Geometry: final body of the model. Coordinates: model frame, mm. A direction names the side the tool comes from. Give positions to 0.01 mm unless a question says otherwise; leave off trailing zeros. Answer as a JSON object with one key per item and string values. Group by question number.
(1) Material intervals for probe 1 along Z at (x, y) = (24.5, 5); probe 2 along Z at (x, y) = (31.5, 4); probe 3 along Y at (x, z) = (4, 50.5), sorted ascending.
(2) Set-up query: faces 1 (the face through (-1, 0, 6.35)), 2 (the face through (38.1, 0, 66)). Return all of +Z, -Z, +X, -X, +Y, -Y with unobstructed straight access to the full face (end or side cutting, diameter ignored); none if empty.
(3) Contact query for flat-ended pins moving along their axis: pin 1 Ø6 at (y, z) = (-5, 24) entering from -X; pin 2 Ø1.5 at (x, y) = (9.5, -3) entering from +Z; pin 3 Ø2 at (x, y) = (10, -1.5) entering from +Z. Output: stop coordinate, or through.
from build123d import *

# Parameters (mm, degrees)
F1_DEPTH = 6.35
F2_R     = 5.08


with BuildPart() as f1:
    # F0 (on Front) → F1 (new body, symmetric)
    with BuildSketch(Plane.XZ):
        with BuildLine():
            Line((-63.5, 6.35), (63.5, 6.35))
            add(Edge.make_bspline(
                [(63.5, 6.35), (-38.796838, 20.9835), (10.021353, 59.327461), (38.1, 59.931301)],
                knots=[0, 0, 0, 0, 59.296845, 59.296845, 59.296845, 59.296845], degree=3))
            Line((38.1, 59.931301), (38.1, 72.631301))
            add(Edge.make_bspline(
                [(-63.5, 6.35), (-62.346671, 26.418077), (-1.330229, 72.954319), (38.1, 72.631301)],
                knots=[0, 0, 0, 0, 121.308577, 121.308577, 121.308577, 121.308577], degree=3))
        make_face()
    extrude(amount=F1_DEPTH, both=True)

    # F2
    f2_edges = [f1.edges().sort_by_distance(p)[0] for p in [
        (-20.792679, -6.35, 51.301252),
        (-20.792679, 6.35, 51.301252),
        (7.139577, 6.35, 24.662786),
        (7.139577, -6.35, 24.662786),
    ]]
    fillet(f2_edges, radius=F2_R)


solid = f1.part
Answer list:
{
 "1": {"probe 1": "6.35 to 13.5, 58.99 to 69.49", "probe 2": "6.35 to 12.11, 59.99 to 71.48", "probe 3": "-6.34 to 6.34"},
 "2": {"face 1": "-Z, +X, -X, +Y, -Y", "face 2": "+Z, +X, +Y, -Y"},
 "3": {"pin 1": "x = -55.3", "pin 2": "z = 66.75", "pin 3": "z = 67.25"}
}
